```python
from build123d import *

# Parameters (mm, degrees)
SKETCH_1_W           = 120
SKETCH_1_H           = 110
EXTRUDE_2_DEPTH      = 120
SKETCH_2_W           = 118
SKETCH_2_H           = 118
CUT_EXTRUDE_1_DEPTH  = 109
SKETCH_5_W           = 109
SKETCH_5_H           = 118
CUT_EXTRUDE_2_DEPTH  = 109
SKETCH_6_W           = 119
SKETCH_6_H           = 109
CUT_EXTRUDE_3_DEPTH  = 109
SKETCH_7_W           = 1
SKETCH_7_H           = 109
EXTRUDE_3_DEPTH      = 119
SKETCH_8_W           = 119
SKETCH_8_H           = 1
EXTRUDE_5_DEPTH      = 119
SKETCH_9_W           = 36
SKETCH_9_H           = 10
CUT_EXTRUDE_4_DEPTH  = 39
SKETCH_11_W          = 36
SKETCH_11_H          = 10
CUT_EXTRUDE_5_DEPTH  = 39
SKETCH_12_W          = 36
SKETCH_12_H          = 99
EXTRUDE_6_DEPTH      = 30
CUT_EXTRUDE_6_DEPTH  = 100
SKETCH_14_W          = 36
SKETCH_14_H          = 99
EXTRUDE_7_DEPTH      = 30
CUT_EXTRUDE_7_DEPTH  = 100
EXTRUDE_9_DEPTH      = 20
CUT_EXTRUDE_8_DEPTH  = 10
CUT_EXTRUDE_9_DEPTH  = 10
SKETCH_22_W          = 0.925592825
SKETCH_22_H          = 19.270027161
EXTRUDE_10_DEPTH     = 30
CUT_EXTRUDE_14_DEPTH = 5
SKETCH_27_R          = 8
EXTRUDE_14_DEPTH     = 40
SKETCH_29_R          = 5.381413495
CUT_EXTRUDE_15_DEPTH = 5
SKETCH_30_R          = 1.016249725
EXTRUDE_15_DEPTH     = 10
EXTRUDE_16_DEPTH     = 3
SKETCH_32_W          = 44.189123475
SKETCH_32_H          = 49.118532685
EXTRUDE_17_DEPTH     = 2
SKETCH_33_W          = 59
SKETCH_33_H          = 119
CUT_EXTRUDE_16_DEPTH = 10


with BuildPart() as part:
    # 스케치1 → 보스-돌출2 (new body)
    with BuildSketch(Plane(origin=(0, 0, 0), x_dir=(1, 0, 0), z_dir=(0, 1, 0))):
        Rectangle(SKETCH_1_W, SKETCH_1_H)
    extrude(amount=EXTRUDE_2_DEPTH)

    # 스케치2 → 컷-돌출1 (cut)
    with BuildSketch(Plane.XY.offset(55)):
        with Locations((0, 60)):
            Rectangle(SKETCH_2_W, SKETCH_2_H)
    extrude(amount=-CUT_EXTRUDE_1_DEPTH, mode=Mode.SUBTRACT)

    # 스케치5 → 컷-돌출2 (cut)
    with BuildSketch(Plane.ZY.offset(60)):
        with Locations((0.5, 60)):
            Rectangle(SKETCH_5_W, SKETCH_5_H)
    extrude(amount=-CUT_EXTRUDE_2_DEPTH, mode=Mode.SUBTRACT)

    # 스케치6 → 컷-돌출3 (cut)
    with BuildSketch(Plane(origin=(0, 120, 0), x_dir=(1, 0, 0), z_dir=(0, 1, 0))):
        with Locations((-0.5, -0.5)):
            Rectangle(SKETCH_6_W, SKETCH_6_H)
    extrude(amount=-CUT_EXTRUDE_3_DEPTH, mode=Mode.SUBTRACT)

    # 스케치7 → 보스-돌출3 (add)
    with BuildSketch(Plane(origin=(0, 1, 0), x_dir=(1, 0, 0), z_dir=(0, 1, 0))):
        with Locations((-0.5, -0.5)):
            Rectangle(SKETCH_7_W, SKETCH_7_H)
    extrude(amount=EXTRUDE_3_DEPTH)

    # 스케치8 → 보스-돌출5 (add)
    with BuildSketch(Plane(origin=(0, 1, 0), x_dir=(1, 0, 0), z_dir=(0, 1, 0))):
        with Locations((-0.5, -0.5)):
            Rectangle(SKETCH_8_W, SKETCH_8_H)
    extrude(amount=EXTRUDE_5_DEPTH)

    # 스케치9 → 컷-돌출4 (cut)
    with BuildSketch(Plane.ZY.offset(1)):
        with Locations((-26, 115)):
            Rectangle(SKETCH_9_W, SKETCH_9_H)
        with Locations((-26, 6)):
            Rectangle(SKETCH_9_W, SKETCH_9_H)
    extrude(amount=-CUT_EXTRUDE_4_DEPTH, mode=Mode.SUBTRACT)

    # 스케치11 → 컷-돌출5 (cut)
    with BuildSketch(Plane.ZY.offset(1)):
        with Locations((29, 115)):
            Rectangle(SKETCH_11_W, SKETCH_11_H)
        with Locations((29, 6)):
            Rectangle(SKETCH_11_W, SKETCH_11_H)
    extrude(amount=-CUT_EXTRUDE_5_DEPTH, mode=Mode.SUBTRACT)

    # 스케치12 → 보스-돌출6 (add)
    with BuildSketch(Plane.ZY.offset(1)):
        with Locations((-26, 60.5)):
            Rectangle(SKETCH_12_W, SKETCH_12_H)
    extrude(amount=EXTRUDE_6_DEPTH)

    # 스케치13 → 컷-돌출6 (cut)
    with BuildSketch(Plane(origin=(0, 110, 0), x_dir=(1, 0, 0), z_dir=(0, 1, 0))):
        Polygon((-1, 44), (-16, 8), (-31, 8), (-31, 44), align=None)
        Polygon((0, 44), (-15, 8), (0, 8), align=None)
    extrude(amount=-CUT_EXTRUDE_6_DEPTH, mode=Mode.SUBTRACT)

    # 스케치14 → 보스-돌출7 (add)
    with BuildSketch(Plane.ZY.offset(1)):
        with Locations((29, 60.5)):
            Rectangle(SKETCH_14_W, SKETCH_14_H)
    extrude(amount=EXTRUDE_7_DEPTH)

    # 스케치15 → 컷-돌출7 (cut)
    with BuildSketch(Plane(origin=(0, 110, 0), x_dir=(1, 0, 0), z_dir=(0, 1, 0))):
        Polygon((-1, -11), (-16, -47), (-31, -47), (-31, -11), align=None)
        Polygon((0, -11), (-15, -47), (0, -47), align=None)
    extrude(amount=-CUT_EXTRUDE_7_DEPTH, mode=Mode.SUBTRACT)

    # 스케치16 → 보스-돌출9 (add)
    with BuildSketch(Plane(origin=(0, 1, 0), x_dir=(1, 0, 0), z_dir=(0, 1, 0))):
        with BuildLine():
            Line((48.146914235, -39.33942453), (23.856416777, -39.33942453))
            ThreePointArc((23.856416777, -39.33942453), (13.856416777, -29.33942453), (23.856416777, -19.33942453))
            Line((23.856416777, -19.33942453), (48.146914235, -19.33942453))
            ThreePointArc((48.146914235, -19.33942453), (58.146914235, -29.33942453), (48.146914235, -39.33942453))
        make_face()
        with BuildLine():
            Line((48.146914235, 38.33942453), (23.856416777, 38.33942453))
            ThreePointArc((23.856416777, 38.33942453), (13.856416777, 28.33942453), (23.856416777, 18.33942453))
            Line((23.856416777, 18.33942453), (48.146914235, 18.33942453))
            ThreePointArc((48.146914235, 18.33942453), (58.146914235, 28.33942453), (48.146914235, 38.33942453))
        make_face()
    extrude(amount=EXTRUDE_9_DEPTH)

    # 스케치17 → 컷-돌출8 (cut)
    with BuildSketch(Plane(origin=(0, 21, 0), x_dir=(1, 0, 0), z_dir=(0, 1, 0))):
        with BuildLine():
            Line((23.856416777, -21.474798149), (42.567688879, -21.474798149))
            ThreePointArc((42.567688879, -21.474798149), (50.43231526, -29.33942453), (42.567688879, -37.204050911))
            Line((42.567688879, -37.204050911), (23.856416777, -37.204050911))
            ThreePointArc((23.856416777, -37.204050911), (15.991790397, -29.33942453), (23.856416777, -21.474798149))
        make_face()
        with BuildLine():
            Line((23.856416777, 20.474798149), (42.567688879, 20.474798149))
            ThreePointArc((42.567688879, 20.474798149), (50.43231526, 28.33942453), (42.567688879, 36.204050911))
            Line((42.567688879, 36.204050911), (23.856416777, 36.204050911))
            ThreePointArc((23.856416777, 36.204050911), (15.991790397, 28.33942453), (23.856416777, 20.474798149))
        make_face()
    extrude(amount=-CUT_EXTRUDE_8_DEPTH, mode=Mode.SUBTRACT)

    # 스케치19 → 컷-돌출9 (cut)
    with BuildSketch(Plane(origin=(0, 11, 0), x_dir=(1, 0, 0), z_dir=(0, 1, 0))):
        with BuildLine():
            Line((39.6013509, 31.146236018), (44.272476327, 31.146236018))
            ThreePointArc((44.272476327, 31.146236018), (46.906569613, 28.512142732), (44.272476327, 25.878049447))
            Line((44.272476327, 25.878049447), (39.6013509, 25.878049447))
            ThreePointArc((39.6013509, 25.878049447), (36.967257615, 28.512142732), (39.6013509, 31.146236018))
        make_face()
        with BuildLine():
            Line((39.6013509, -32.146236018), (44.272476327, -32.146236018))
            ThreePointArc((44.272476327, -32.146236018), (46.906569613, -29.512142732), (44.272476327, -26.878049447))
            Line((44.272476327, -26.878049447), (39.6013509, -26.878049447))
            ThreePointArc((39.6013509, -26.878049447), (36.967257615, -29.512142732), (39.6013509, -32.146236018))
        make_face()
    extrude(amount=-CUT_EXTRUDE_9_DEPTH, mode=Mode.SUBTRACT)

    # 스케치22 → 보스-돌출10 (add)
    with BuildSketch(Plane(origin=(0, 21, 0), x_dir=(1, 0, 0), z_dir=(0, 1, 0))):
        with Locations((51.210576598, -29.360263905)):
            Rectangle(SKETCH_22_W, SKETCH_22_H)
        with Locations((51.210576598, 28.360263905)):
            Rectangle(SKETCH_22_W, SKETCH_22_H)
    extrude(amount=EXTRUDE_10_DEPTH)

    # 스케치26 → 컷-돌출14 (cut)
    with BuildSketch(Plane.ZY.offset(-50.747780185)):
        with BuildLine():
            Line((19.725250325, 51), (19.725250325, 42.862531911))
            ThreePointArc((19.725250325, 42.862531911), (29.360263905, 50.947462847), (38.995277486, 42.862531911))
            Line((38.995277486, 42.862531911), (38.995277486, 51))
            Line((38.995277486, 51), (19.725250325, 51))
        make_face()
        with BuildLine():
            Line((-38.143872213, 41.16385454), (-38.143872213, 57.416257422))
            Line((-38.143872213, 57.416257422), (-18.576655598, 57.416257422))
            Line((-18.576655598, 57.416257422), (-18.576655598, 41.16385454))
            ThreePointArc((-18.576655598, 41.16385454), (-28.360263905, 50.947462847), (-38.143872213, 41.16385454))
        make_face()
    extrude(amount=-CUT_EXTRUDE_14_DEPTH, mode=Mode.SUBTRACT)

    # 스케치27 → 보스-돌출14 (add)
    with BuildSketch(Plane(origin=(0, 1, 0), x_dir=(1, 0, 0), z_dir=(0, 1, 0))):
        with Locations(Location((-30.5, 44, 0), (0, 0, 90))):
            Circle(SKETCH_27_R)
    extrude(amount=EXTRUDE_14_DEPTH)

    # 스케치29 → 컷-돌출15 (cut)
    with BuildSketch(Plane(origin=(0, 41, 0), x_dir=(1, 0, 0), z_dir=(0, 1, 0))):
        with Locations(Location((-30.5, 42.18650453, 0), (0, 0, 270))):
            Circle(SKETCH_29_R)
    extrude(amount=-CUT_EXTRUDE_15_DEPTH, mode=Mode.SUBTRACT)

    # 스케치30 → 보스-돌출15 (add)
    with BuildSketch(Plane(origin=(0, 41, 0), x_dir=(1, 0, 0), z_dir=(0, 1, 0))):
        with Locations(Location((-30.5, 49.674732838, 0), (0, 0, 270))):
            Circle(SKETCH_30_R)
    extrude(amount=EXTRUDE_15_DEPTH)

    # 스케치31 → 보스-돌출16 (add)
    with BuildSketch(Plane(origin=(0, 51, 0), x_dir=(1, 0, 0), z_dir=(0, 1, 0))):
        with BuildLine():
            Line((-29.503658446, 49.674732838), (-29.503658446, 46.055904325))
            ThreePointArc((-29.503658446, 46.055904325), (-30.5, 45.059562771), (-31.496341554, 46.055904325))
            Line((-31.496341554, 46.055904325), (-31.496341554, 49.674732838))
            ThreePointArc((-31.496341554, 49.674732838), (-30.5, 50.671074391), (-29.503658446, 49.674732838))
        make_face()
    extrude(amount=EXTRUDE_16_DEPTH)

    # 스케치32 → 보스-돌출17 (add)
    with BuildSketch(Plane.XY.offset(-54)):
        with Locations((-25.626680732, 80.311397781)):
            Rectangle(SKETCH_32_W, SKETCH_32_H)
    extrude(amount=EXTRUDE_17_DEPTH)

    # 스케치33 → 컷-돌출16 (cut)
    with BuildSketch(Plane.XY.offset(1)):
        with Locations((-30.5, 60.5)):
            Rectangle(SKETCH_33_W, SKETCH_33_H)
    extrude(amount=-CUT_EXTRUDE_16_DEPTH, mode=Mode.SUBTRACT)


solid = part.part
```
Here's how the part is built. I have some questions about the finished solid (model axes, mm). A direction names the side the tool comes from. Coordinates: 2 decimals unless noted, no trailing zeros. Write each loop counter-clockwise with the first axis right and the second up, starting at its lowest first coordinate (ties: lowest second). Pieces come first, ordered by that corner, then holes. Notation, with made-up numbers: (53.25, 54) -> (85.25, 54) arc R31 ccw to (85.25, 86) -> close; hole circle Ø9 at (82.25, 88.25). An arc over 180 degrees is marked (long way). Use a Markdown table: item, result. Add a question column.
(1) I'm going to push flat-ended pins straight in: P1, Ø5, axis at x = 15, y = 40, coming from the +Z side; P2, Ø4.5, axis at x = 30.5, z = 26, coming from the +Y side; P3, Ø16, axis at x = 32.5, z = -27, coming from the +Y side. Where does each tip first touch, or does it pass through?
(2) If we section it at A-A, the plane z = 5.5: Write out the boundary of the cut face in (x, y), and give its area (3 significant figures).
(3) If we section it at C-C, the plane z = -40: Write out the boundary of the cut face in (x, y).
(4) Please list where these lines run through material, in increasing order: line 1 (Z direction, x = -30, y = 39); line 2 (X direction, y = 66, z = -50); line 3 (Z direction, x = -8, y = 25.5).
(5) We'd pull the mould along X, two halves only. Please class faces 1 (the flat face through (-7.8, 110, -26.6)), 2 (the flat face through (60, 59, 1)), 3 (the cylindrical face through (15.994, 16.07, -28.512)): +X half, -X half, draft (parallel to the pull), parting line (faces both ways), or undercut.
(6) If we section it at D-D, the plane x = 10: Write out the boundary of the cut face in (y, z), and give its area (3 significant figures).
(7) For faces 4 (the flat face through (-1, 59, -55)), 5 (the flat face through (51.673, 36, 29)), 6 (the flat face through (-1, 60, 2)), 7 (the cylindrical face through (50.43, 16.07, 29.17)), which set-ups out of +Z, -Z, +X, -X, +Y, -Y let a thin tool reach every point of the face, with its end or its side?
Outcome:
| question | item | result |
|---|---|---|
| 1 | P1 | stops at z = 1 |
| 1 | P2 | stops at y = 11 |
| 1 | P3 | stops at y = 21 |
| 2 | outline | (-60, 0) -> (60, 0) -> (60, 120) -> (59, 120) -> (59, 1) -> (0, 1) -> (0, 120) -> (-1, 120) -> (-1, 1) -> (-60, 1) -> close |
| 2 | area | 358 mm^2 |
| 3 | outline | (-60, 0) -> (60, 0) -> (60, 120) -> (59, 120) -> (59, 1) -> (-23.57, 1) -> (-23.57, 41) -> (-25.58, 41) -> (-25.58, 36) -> (-35.42, 36) -> (-35.42, 41) -> (-37.43, 41) -> (-37.43, 1) -> (-60, 1) -> close; (-2.67, 11) -> (-1.67, 11) -> (-1.67, 110) -> (-2.67, 110) -> close |
| 4 | line 1 | z = -55 to -54, -51.98 to -47.54, -36.83 to -36.02 |
| 4 | line 2 | x = -1 to 0, 59 to 60 |
| 4 | line 3 | z = -55 to -54, -27.2 to -24.8, 27.8 to 30.2 |
| 5 | face 1 | draft |
| 5 | face 2 | +X half |
| 5 | face 3 | undercut |
| 6 | outline | (0, -55) -> (120, -55) -> (120, -54) -> (1, -54) -> (1, 0) -> (120, 0) -> (120, 1) -> (1, 1) -> (1, 55) -> (0, 55) -> close |
| 6 | area | 348 mm^2 |
| 7 | face 4 | -Z, +X, -X, +Y, -Y |
| 7 | face 5 | +Z, +Y |
| 7 | face 6 | -X, +Y |
| 7 | face 7 | +Y |
